from build123d import *

# Parameters (mm, degrees)
SKETCH2_W           = 38
SKETCH2_H           = 38
SKETCH3_W           = 30
SKETCH3_H           = 30
SKETCH4_R           = 4
CUT_EXTRUDE1_DEPTH  = 39
SWEEP2_PROFILE_R    = 2.5
CUT_EXTRUDE2_DEPTH  = 39
BOSS_EXTRUDE1_DEPTH = 38
SKETCH22_W          = 30
SKETCH22_H          = 30
CUT_EXTRUDE3_DEPTH  = 835.558043559
CUT_EXTRUDE4_DEPTH  = 39
CUT_EXTRUDE5_DEPTH  = 39
BOSS_EXTRUDE2_REACH = 40


with BuildPart() as part:
    # Sweep1: sweep along a path in Sketch1
    with BuildLine(Plane(origin=(0, 0, 0), x_dir=(1, 0, 0), z_dir=(0, 1, 0))) as sweep1_path:
        Line((0, 0), (-762.63683242, 0))
    # Sketch2 → Sweep1 (sweep)
    with BuildSketch(Plane(origin=(0, 0, 0), x_dir=(0, 0, -1), z_dir=(1, 0, 0))):
        Rectangle(SKETCH2_W, SKETCH2_H)
    sweep(path=sweep1_path.line)

    # Cut-Sweep1: sweep along a path in Sketch1_2
    with BuildLine(Plane(origin=(0, 0, 0), x_dir=(1, 0, 0), z_dir=(0, 1, 0))) as cut_sweep1_path:
        Line((0, 0), (-762.63683242, 0))
    # Sketch3 → Cut-Sweep1 (sweep, cut)
    with BuildSketch(Plane(origin=(0, 0, 0), x_dir=(0, 0, -1), z_dir=(1, 0, 0))):
        Rectangle(SKETCH3_W, SKETCH3_H)
    sweep(path=cut_sweep1_path.line, mode=Mode.SUBTRACT)

    # Sketch4 → Cut-Extrude1 (cut, through all)
    with BuildSketch(Plane(origin=(0, 19, 0), x_dir=(1, 0, 0), z_dir=(0, 1, 0))):
        with Locations((-212.63683242, 0)):
            Circle(SKETCH4_R)
    extrude(amount=-CUT_EXTRUDE1_DEPTH, mode=Mode.SUBTRACT)

    # Sweep2: sweep along a path in Sketch5
    with BuildLine(Plane.ZY.offset(747.63683242)) as sweep2_path:
        Line((-19, 0), (-26.570946825, 0))
        ThreePointArc((-26.570946825, 0), (-29.503401087, 0.950220747), (-31.321263798, 3.4397152))
        ThreePointArc((-31.321263798, 3.4397152), (-51.969366005, 0.135523131), (-31.321263798, -3.168668939))
    # Sweep2 profile (on start of the path) → Sweep2 (sweep)
    with BuildSketch(Plane(origin=(-747.63683242, 0, -19), x_dir=(0, -1, 0), z_dir=(0, 0, -1))):
        Circle(SWEEP2_PROFILE_R)
    sweep(path=sweep2_path.line)

    # Sketch16 → Cut-Extrude2 (cut, through all)
    with BuildSketch(Plane(origin=(0, 19, 0), x_dir=(1, 0, 0), z_dir=(0, 1, 0))):
        Polygon((0, -19), (0, 19), (-71.907398101, -19), align=None)
    extrude(amount=-CUT_EXTRUDE2_DEPTH, mode=Mode.SUBTRACT)

    # Sketch17 → Boss-Extrude1 (add)
    with BuildSketch(Plane(origin=(0, 19, 0), x_dir=(1, 0, 0), z_dir=(0, 1, 0))):
        Polygon((-71.907398101, -19), (0, -19), (71.921211139, 19), (0, 19), align=None)
    extrude(amount=-BOSS_EXTRUDE1_DEPTH)

    # Sketch22 → Cut-Extrude3 (cut, through all)
    with BuildSketch(Plane.ZY.offset(762.63683242)):
        Rectangle(SKETCH22_W, SKETCH22_H)
    extrude(amount=-CUT_EXTRUDE3_DEPTH, mode=Mode.SUBTRACT)

    # Sketch23 → Cut-Extrude4 (cut, through all)
    with BuildSketch(Plane(origin=(0, 19, 0), x_dir=(1, 0, 0), z_dir=(0, 1, 0))):
        Polygon((14.258492684, 0), (-32.20683242, -19), (0, -19), (71.921211139, 19), (60.723817789, 19), align=None)
    extrude(amount=-CUT_EXTRUDE4_DEPTH, mode=Mode.SUBTRACT)

    # Sketch24 → Cut-Extrude5 (cut, through all)
    with BuildSketch(Plane(origin=(0, 19, 0), x_dir=(1, 0, 0), z_dir=(0, 1, 0))):
        Polygon((-78.672157524, -19), (14.258492684, 19), (60.723817789, 19), (-32.20683242, -19), align=None)
    extrude(amount=-CUT_EXTRUDE5_DEPTH, mode=Mode.SUBTRACT)

    # Sketch25 → Boss-Extrude2 (add, up to next)
    with BuildSketch(Plane(origin=(0, 19, 0), x_dir=(1, 0, 0), z_dir=(0, 1, 0)), mode=Mode.PRIVATE) as boss_extrude2_sk1:
        Polygon((3.690100071, 19), (-89.240550137, -19), (-78.672157524, -19), (14.258492684, 19), align=None)
    boss_extrude2_tool1 = extrude(boss_extrude2_sk1.sketch, amount=-BOSS_EXTRUDE2_REACH, mode=Mode.PRIVATE) - part.part
    add(boss_extrude2_tool1.solids().sort_by_distance((-37.491029, 19, 0))[0])


solid = part.part
Input: part model. Units: mm. Frame: model coordinates. A direction names the side the tool comes from. Give positions to 0.01 mm unless a question says otherwise; leave off trailing zeros. Order: outer loops, then holes, each group sorted by start corner. A loop starts at its lowest first (then second) coordinate and runs counter-clockwise, first axis right, second up. Notation, with made-up numbers: M -38.75,87 L 12.25,87 A28 ccw 12.25,116 Z; hole C -17.5,-13 d3. An arc over 180 degrees is marked long. Answer as a JSON object with one key per item and string values.
1. Pull-direction query (Y, two-part tool) for faces 3 (the flat face through (-390, 15, 0)), 4 (the flat face through (-425, 0, 19)), 5 (the flat face through (-380, -19, 0)); classes: +Y half, -Y half, draft (parallel to the pull), parting line (faces both ways), or undercut.
Result sheet:
{"face 3": "undercut", "face 4": "draft", "face 5": "-Y half"}
2. Reachability of faces 1 (the flat face through (-426, 0, 15)), 2 (the flat face through (-762.637, 0, 17)) from +Z, -Z, +X, -X, +Y, -Y: full face, straight path, thin tool, end or side. Return the list, or none.
Result sheet:
{"face 1": "-X", "face 2": "+Z, -Z, -X, +Y, -Y"}
3. Ray query, line 1 (Z direction, x = -222, y = 4); line 2 (X direction, y = -17, z = -2). Return the intervals inside material, ascending. Write a range as [from, to].
Result sheet:
{"line 1": "[-19, -15], [15, 19]", "line 2": "[-762.64, -216.1], [-209.17, -27.32]"}
4. First-contact query: P1, Ø19, axis at x = -180, y = 0.5, coming from the -Z side; P2, Ø9, axis at x = -212.64, z = 0, coming from the +Y side; P3, Ø6.5, axis at x = -212.64, z = 0, coming from the +Y side; P4, Ø1.5, axis at y = -8, z = -33, coming from the -X side. Flat tips, straight axial feed; report the tip coordinate or a pass-through.
Result sheet:
{"P1": "z = -19", "P2": "y = 19", "P3": "through", "P4": "x = -750.11"}
5. Cut plane A-A, the plane x = -715.5. Output: boundary loops of the cut face in (y, z).
Result sheet:
{"outline": "M -19,-19 L 19,-19 L 19,19 L -19,19 Z; hole M -15,-15 L 15,-15 L 15,15 L -15,15 Z"}
